Autodesk Inventor part; units mm, degrees
ref_plane "YZ Plane" through (0, 0, 0) normal (1, 0, 0) x (0, 1, 0)
ref_plane "XZ Plane" through (0, 0, 0) normal (0, 1, 0) x (-1, 0, 0)
ref_plane "XY Plane" through (0, 0, 0) normal (0, 0, 1) x (1, 0, 0)
sketch "Sketch1" plane through (0, 0, 0) normal (0, 0, 1) x (1, 0, 0)
  line L0 (0, 0) -> (0, 50)
  line L1 (0, 50) -> (50, 50)
  line L2 (50, 50) -> (50, 100)
  line L3 (50, 100) -> (58, 100)
  line L4 (58, 100) -> (58, 42)
  line L5 (58, 42) -> (8, 42)
  line L6 (8, 42) -> (8, 0)
  line L7 (8, 0) -> (0, 0)
  dimension "d0" = 50
  dimension "d1" = 50
  dimension "d2" = 50
  dimension "d3" = 8
  dimension "d4" = 58
  dimension "d6" = 50
extrude "Extrusion1" add sketch "Sketch1" along normal blind 25
sketch "Sketch2" plane through (58, 42, 0) normal (1, 0, 0) x (0, 0, -1)
  circle A0 centre (-12.5, 50) radius 2.75
  line L0 (0, 58) -> (-25, 58)
  line L1 (-25, 0) -> (-25, 58)
  point P0 (0, -42)
  dimension "d9" = 5.5
  dimension "d10" = 8
  dimension "d11" = 12.5
extrude "Extrusion2" cut sketch "Sketch2" against normal blind 25
sketch "Sketch3" plane through (8, 0, 0) normal (1, 0, 0) x (0, 0, -1)
  point P0 (0, 0)
sketch "Sketch4" plane through (8, 0, 0) normal (1, 0, 0) x (0, 0, -1)
  circle A0 centre (-12.5, 21) radius 3.25
  line L0 (0, 42) -> (-25, 42)
  line L1 (0, 0) -> (0, 42)
  dimension "d26" = 21
  dimension "d27" = 6.5
  dimension "d28" = 12.5
extrude "Extrusion3" cut sketch "Sketch4" against normal blind 25
sketch "Sketch5" plane through (58, 42, 0) normal (1, 0, 0) x (0, 0, -1)
  circle A0 centre (-12.5, 38.2531) radius 2.75
  line L0 (0, 0) -> (0, 58)
  circle A1 centre (-12.5, 24.9243) radius 2.75
  line L1 (-15.25, 38.2531) -> (-15.25, 24.9243)
  line L2 (-9.75, 38.2531) -> (-9.75, 24.9243)
  point P0 (0, -42)
  dimension "d31" = 5.5
  dimension "d32" = 9.75
  dimension "d33" = 5.5
extrude "Extrusion4" cut sketch "Sketch5" against normal blind 58
equation "\"d34\" = d4"
properties part number "CoilBracketMount"
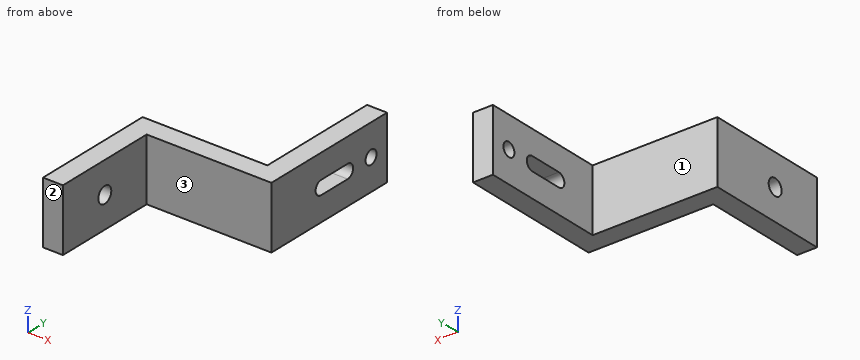
Could you check a few things on this model? Use its own coordinates, in mm. Face numbers are marked on the shaded views. A direction names the side the tool comes from. Round coordinates to 2 decimals unless told otherwise and drop trailing zeros. Write each loop counter-clockwise with the first axis right and the second up, starting at its lowest first coordinate (ties: lowest second). Pieces come first, ordered by that corner, then holes. Notation, with made-up numbers: M -16,32.5 L 21,32.5 A24 ccw 21,52.5 Z; hole C 30.25,2 d10. An arc over 180 degrees is marked long. Write each question's results on one line, items separated by ' | '. Start each with the question number.
1. Imagine slicing it at A-A on y = 92. List the corners of the cut face in (x, z) for me, and give its area (3 significant figures).
2. Imagine slicing it at C-C on z = 19. List the corners of the cut face in (x, y) for me.
3. Imagine slicing it at D-D on y = 21. List the corners of the cut face in (x, z) for me.
4. I'm going to push flat-ended pins straight in: pin 1 Ø6 at (y, z) = (21, 12.5) entering from +X; pin 2 Ø6 at (x, z) = (9.5, 19.5) entering from -Y; pin 3 Ø12.5 at (y, z) = (80, 9) entering from -X; pin 4 Ø12.5 at (x, z) = (33.5, 15) entering from +Y. Where does each tip first touch, or does it pass through?
5. I need wall thicknesses on L1, parallel to Y at x = 52, z = 12.5; L2, parallel to Y at x = 1.5, z = 12.5; L3, parallel to X at y = 12.5, z = 22. Which ranges of each line are inside material? Lowest first, please. Write a range as from..to.
6. Imagine slicing it at B-B on z = 12.5. List the corners of the cut face in (x, y) for me.
7. On a 3-axis mill with a long thin cutter (end or side, diameter ignored), from which of +Z, -Z, +X, -X, +Y, -Y can I reach the whole of each face in a straight line? I mean the marked faces 1, 2 and 3. Say none if no direction works.
Result sheet:
1) outline: M 50,0 L 58,0 L 58,9.75 L 50,9.75 Z; M 50,15.25 L 58,15.25 L 58,25 L 50,25 Z | area: 156 mm^2
2) outline: M 0,0 L 8,0 L 8,42 L 58,42 L 58,100 L 50,100 L 50,50 L 0,50 Z
3) outline: M 0,0 L 8,0 L 8,9.25 L 0,9.25 Z; M 0,15.75 L 8,15.75 L 8,25 L 0,25 Z
4) pin 1: passes through | pin 2: stops at y = 0 | pin 3: stops at x = 50 | pin 4: stops at y = 50
5) L1: y = 42..64.17, 83..89.25, 94.75..100 | L2: y = 0..17.75, 24.25..50 | L3: x = 0..8
6) outline: M 0,0 L 8,0 L 8,17.75 L 0,17.75 Z; M 0,24.25 L 8,24.25 L 8,42 L 58,42 L 58,64.17 L 50,64.17 L 50,50 L 0,50 Z; M 50,83 L 58,83 L 58,89.25 L 50,89.25 Z; M 50,94.75 L 58,94.75 L 58,100 L 50,100 Z
7) face 1: +Z, -Z, -X, +Y | face 2: +Z, -Z, +X, -X, -Y | face 3: +Z, -Z, +X, -Y
